from build123d import *

# Parameters (mm, degrees)
SKETCH_1_W          = 50
SKETCH_1_H          = 50
SKETCH_1_R          = 1.55
SKETCH_1_R_2        = 6.05
EXTRUDE_1_DEPTH     = 3
FILLET_1_R          = 5
SKETCH_2_R          = 1.55
CUT_EXTRUDE_1_DEPTH = 36.482389998


with BuildPart() as part:
    # ｽｹｯﾁ1 → ﾎﾞｽ - 押し出し1 (new body)
    with BuildSketch(Plane.XY):
        Rectangle(SKETCH_1_W, SKETCH_1_H)
        with Locations((-20, 20)):
            Circle(SKETCH_1_R, mode=Mode.SUBTRACT)
        with Locations((20, 20)):
            Circle(SKETCH_1_R, mode=Mode.SUBTRACT)
        with Locations((20, -20)):
            Circle(SKETCH_1_R, mode=Mode.SUBTRACT)
        with Locations((-20, -20)):
            Circle(SKETCH_1_R, mode=Mode.SUBTRACT)
        Circle(SKETCH_1_R_2, mode=Mode.SUBTRACT)
        with Locations((-9, 0)):
            Circle(SKETCH_1_R, mode=Mode.SUBTRACT)
        with Locations(Location((9, 0, 0), (0, 0, 180))):
            Circle(SKETCH_1_R, mode=Mode.SUBTRACT)
    extrude(amount=EXTRUDE_1_DEPTH)

    # ﾌｨﾚｯﾄ1
    fillet_1_edges = [part.edges().sort_by_distance(p)[0] for p in [
        (25, -25, 1.5),
        (-25, -25, 1.5),
        (-25, 25, 1.5),
        (25, 25, 1.5),
    ]]
    fillet(fillet_1_edges, radius=FILLET_1_R)

    # ｽｹｯﾁ2 → ｶｯﾄ - 押し出し1 (cut, through all)
    with BuildSketch(Plane.XY.offset(3)):
        with Locations((-10, 20)):
            Circle(SKETCH_2_R)
        with Locations(Location((10, 20, 0), (0, 0, 180))):
            Circle(SKETCH_2_R)
        with Locations((10, -20)):
            Circle(SKETCH_2_R)
        with Locations(Location((-10, -20, 0), (0, 0, 180))):
            Circle(SKETCH_2_R)
    extrude(amount=-CUT_EXTRUDE_1_DEPTH, mode=Mode.SUBTRACT)


solid = part.part
Can you work these out from the model? Positions are in its coordinate system, mm. Coordinates: 2 decimals unless noted, no trailing zeros. Order: outer loops, then holes, each group sorted by start corner. A loop starts at its lowest first (then second) coordinate and runs counter-clockwise, first axis right, second up. Notation, with made-up numbers: M -28.5,34 L 28.5,34 A20 ccw 28.5,51 Z; hole C 0,69.25 d8. An arc over 180 degrees is marked long. Answer as CSV lines item,"result".
(1) I'm going to push flat-ended pins straight in: pin 1 (3.5 mm diameter, centred on x = -20, y = 20, fed in from +Z); pin 2 (1.9 mm diameter, centred on x = 10, y = -20, fed in from +Z). Where does each tip first touch, or does it pass through?
Geometry check:
pin 1,"z = 3"
pin 2,"through"
(2) Suppose I cut it at A-A on x = 0. Please give me the cut outline in (y, z).
Geometry check:
outline,"M -25,0 L -6.05,0 L -6.05,3 L -25,3 Z; M 6.05,0 L 25,0 L 25,3 L 6.05,3 Z"
(3) If we mould it in two halves opening along Y, with no side actions, what happens to faces 1 (the cylindrical face through (-24, 23, 2)), 2 (the cylindrical face through (-20.202, 21.537, 1.479)), 3 (the cylindrical face through (8.17, -1.31, 1.48)), 4 (the cylindrical face through (23, -24, 2))? For each: released by +Y, released by -Y, zero draft, split by the parting line, or undercut.
Geometry check:
face 1,"released by +Y"
face 2,"undercut"
face 3,"undercut"
face 4,"released by -Y"
(4) Please list where these lines run through material, in increasing order: L1, parallel to Y at x = -20, z = 0.55; L2, parallel to Y at x = 9, z = 0.8; L3, parallel to Y at x = 0, z = 1.7.
Geometry check:
L1,"-25 to -21.55, -18.45 to 18.45, 21.55 to 25"
L2,"-25 to -21.18, -18.82 to -1.55, 1.55 to 18.82, 21.18 to 25"
L3,"-25 to -6.05, 6.05 to 25"
(5) Suppose I cut it at B-B on z = 0.5. Count the separate pieces of the cut face and the enclosed holes in it, plus the area to 3 significant figures.
Geometry check:
separate pieces,"1"
enclosed holes,"11"
area,"2,290 mm^2"
